Read the model definition and answer for the solid it produces. Units are mm, in the model's axes. A direction names the side the tool comes from. Coordinates: 2 decimals unless noted, no trailing zeros. Write each loop counter-clockwise with the first axis right and the second up, starting at its lowest first coordinate (ties: lowest second). Pieces come first, ordered by that corner, then holes. Notation, with made-up numbers: (-1, 23) -> (31, 23) arc R34 ccw to (31, 57) -> close; hole circle Ø1 at (37.25, 65.5). An arc over 180 degrees is marked (long way). Return JSON: item names as keys, results as strings.
Autodesk Inventor part; units mm, degrees
ref_plane "CP1_XY" through (0, 0, -77.4) normal (0, 0, -1) x (1, 0, 0)
ref_plane "CP1_YZ" through (0, 0, -77.4) normal (1, 0, 0) x (0, -1, 0)
ref_plane "CP1_ZX" through (0, 0, -77.4) normal (0, -1, 0) x (0, 0, -1)
sketch "Sketch_1" plane through (0, 0, 0) normal (1, 0, 0) x (0, 1, 0)
  line L0 (0, -77.4) -> (0, 0)
  line L1 (0, 0) -> (3, 0)
  line L2 (3, 0) -> (3, -72.4)
  line L3 (3, -72.4) -> (8, -72.4)
  line L4 (8, -72.4) -> (8, -77.4)
  line L5 (8, -77.4) -> (0, -77.4)
  line L6 (0, -77.4) -> (0, 0)
revolve "Revolution1" add sketch "Sketch_1" angle 360 about axis through (0, 0, -77.4) along (0, 0, -1)
sketch "Sketch_2" plane through (0, 0, 0) normal (1, 0, 0) x (0, 1, 0)
  line L0 (0, 0) -> (0, 12)
  line L1 (0, 12) -> (2.3865, 12)
  line L2 (2.3865, 12) -> (3, 11.3865)
  line L3 (3, 11.3865) -> (3, 2.2222)
  line L4 (3, 2.2222) -> (2.0586, 1.2808)
  arc A0 (2.0586, 1.2808) -> (2, 1.1394) centre (2.2, 1.1394) ccw
  line L5 (2, 1.1394) -> (2, 0.2)
  arc A1 (2, 0.2) -> (2.2, 0) centre (2.2, 0.2) ccw
  line L6 (2.2, 0) -> (0, 0)
  line L7 (0, 0) -> (0, 12)
revolve "Revolution2" add sketch "Sketch_2" angle 360 about axis through (0, 0, 0) along (0, 0, -1)
thread "Thread1"
sketch "Sketch_8" plane through (0, 0, 0) normal (0, 0, 1) x (1, 0, 0)
  line L0 (-4.5, 5) -> (-4.5, -5)
  line L1 (-4.5, -5) -> (4.5, -5)
  line L2 (4.5, -5) -> (4.5, 5)
  line L3 (4.5, 5) -> (-4.5, 5)
  line L4 (-2.5, -4) -> (2.5, -4)
  line L5 (2.5, -4) -> (2.5, 4)
  line L6 (2.5, 4) -> (-2.5, 4)
  line L7 (-2.5, 4) -> (-2.5, -4)
extrude "Extrusion1" cut sketch "Sketch_8" against normal blind 3
ref_plane "CP1_XY" through (0, 0, -77.4) normal (0, 0, -1) x (1, 0, 0)
ref_plane "CP1_YZ" through (0, 0, -77.4) normal (1, 0, 0) x (0, -1, 0)
ref_plane "CP1_ZX" through (0, 0, -77.4) normal (0, -1, 0) x (0, 0, -1)
ref_plane "CP_P_XY" through (0, 0, -77.4) normal (0, 0, 1) x (1, 0, 0)
ref_plane "CP_P_YZ" through (0, 0, -77.4) normal (1, 0, 0) x (0, 1, 0)
ref_plane "CP_P_ZX" through (0, 0, -77.4) normal (0, 1, 0) x (0, 0, 1)
ref_plane "CP_PL_XY" through (0, 0, -3) normal (0, 0, 1) x (1, 0, 0)
ref_plane "CP_PL_YZ" through (0, 0, -3) normal (1, 0, 0) x (0, 1, 0)
ref_plane "CP_PL_ZX" through (0, 0, -3) normal (0, 1, 0) x (0, 0, 1)
ref_plane "DIM_ZM_XY" through (0, 3, -150) normal (1, 0, 0) x (0, 0, -1)
ref_plane "DIM_ZM_YZ" through (0, 3, -150) normal (0, 0, -1) x (0, 1, 0)
ref_plane "DIM_ZM_ZX" through (0, 3, -150) normal (0, 1, 0) x (1, 0, 0)
ref_plane "DISC_XY" through (0, 0, 5) normal (0, 0, -1) x (1, 0, 0)
ref_plane "DISC_YZ" through (0, 0, 5) normal (1, 0, 0) x (0, -1, 0)
ref_plane "DISC_ZX" through (0, 0, 5) normal (0, -1, 0) x (0, 0, -1)
ref_plane "NUT_6_10_T_1_XY" through (0, 0, -161) normal (0, 0, 1) x (1, 0, 0)
ref_plane "NUT_6_10_T_1_YZ" through (0, 0, -161) normal (1, 0, 0) x (0, 1, 0)
ref_plane "NUT_6_10_T_1_ZX" through (0, 0, -161) normal (0, 1, 0) x (0, 0, 1)
ref_plane "NUT_6_10_T_2_XY" through (0, 0, -158.8) normal (0, 0, 1) x (1, 0, 0)
ref_plane "NUT_6_10_T_2_YZ" through (0, 0, -158.8) normal (1, 0, 0) x (0, 1, 0)
ref_plane "NUT_6_10_T_2_ZX" through (0, 0, -158.8) normal (0, 1, 0) x (0, 0, 1)
ref_plane "NUT_CP_6_10_1_XY" through (0, 0, 10) normal (0, 0, 1) x (1, 0, 0)
ref_plane "NUT_CP_6_10_1_YZ" through (0, 0, 10) normal (1, 0, 0) x (0, 1, 0)
ref_plane "NUT_CP_6_10_1_ZX" through (0, 0, 10) normal (0, 1, 0) x (0, 0, 1)
ref_plane "NUT_CP_6_10_2_XY" through (0, 0, 7.8) normal (0, 0, 1) x (1, 0, 0)
ref_plane "NUT_CP_6_10_2_YZ" through (0, 0, 7.8) normal (1, 0, 0) x (0, 1, 0)
ref_plane "NUT_CP_6_10_2_ZX" through (0, 0, 7.8) normal (0, 1, 0) x (0, 0, 1)
properties part number "4186566 DPDM-50---(r)" material "Stainless Steel"
1. Flat-ended cylindrical pins translate along their axes: pin 1 Ø0.9 at (y, z) = (0, -2) entering from +X; pin 2 Ø8 at (y, z) = (-1, -3) entering from +X; pin 3 Ø6 at (x, z) = (1, -54) entering from -Y. Find the tip coordinate at first contact, or state that the pin passes through.
Taken from the geometry:
{"pin 1": "stops at x = 2.5", "pin 2": "stops at x = 3", "pin 3": "stops at y = -3"}
2. The part is cut by section D-D (x = -5.75). Determine the outline of the cut face in (y, z), then the cut area to 3 significant figures.
Taken from the geometry:
{"outline": "(-5.56, -77.4) -> (5.56, -77.4) -> (5.56, -72.4) -> (-5.56, -72.4) -> close", "area": "55.6 mm2"}
3. Consider L1, parallel to Z at x = 1.75, y = 3.75; L2, parallel to X at y = 0, z = -9; L3, parallel to X at y = -2, z = -33.5. Determine where each line is inside the solid, lowest interval first.
Taken from the geometry:
{"L1": "z = -77.4 to -72.4", "L2": "x = -3 to 3", "L3": "x = -2.24 to 2.24"}
4. The part is cut by section B-B (x = 0). Determine the outline of the cut face in (y, z), then the cut area to 3 significant figures.
Taken from the geometry:
{"outline": "(-8, -77.4) -> (8, -77.4) -> (8, -72.4) -> (3, -72.4) -> (3, 0) -> (2.2, 0) arc R0.2 cw to (2, 0.2) -> (2, 1.14) arc R0.2 cw to (2.06, 1.28) -> (3, 2.22) -> (3, 11.39) -> (2.39, 12) -> (-2.39, 12) -> (-3, 11.39) -> (-3, 2.22) -> (-2.06, 1.28) arc R0.2 cw to (-2, 1.14) -> (-2, 0.2) arc R0.2 cw to (-2.2, 0) -> (-3, 0) -> (-3, -72.4) -> (-8, -72.4) -> close", "area": "583 mm2"}
5. The part is cut by section A-A (y = 0). Determine the outline of the cut face in (x, z).
Taken from the geometry:
{"outline": "(-8, -77.4) -> (8, -77.4) -> (8, -72.4) -> (3, -72.4) -> (3, -3) -> (2.5, -3) -> (2.5, 0) -> (2.2, 0) arc R0.2 cw to (2, 0.2) -> (2, 1.14) arc R0.2 cw to (2.06, 1.28) -> (3, 2.22) -> (3, 11.39) -> (2.39, 12) -> (-2.39, 12) -> (-3, 11.39) -> (-3, 2.22) -> (-2.06, 1.28) arc R0.2 cw to (-2, 1.14) -> (-2, 0.2) arc R0.2 cw to (-2.2, 0) -> (-2.5, 0) -> (-2.5, -3) -> (-3, -3) -> (-3, -72.4) -> (-8, -72.4) -> close"}
6. For a pull along Z with two mould halves and no side action, classify faces 1 (the face through (-1.952, -0.434, 0.663)), 2 (the face through (0, -3, -37)), 3 (the face through (0, 0, -77.4)) as +Z half, -Z half, draft (parallel to the pull), parting line (faces both ways), or undercut.
Taken from the geometry:
{"face 1": "undercut", "face 2": "draft", "face 3": "-Z half"}
7. A tool of negligible diameter and unlimited length cuts with its end or side. For faces 4 (the face through (0.1, 3.4, -72.4)), 5 (the face through (2.3, 0.6, 0)), 6 (the face through (2.5, 0, -1)), from which of +Z, -Z, +X, -X, +Y, -Y can it reach the whole face along a straight path? Write none if from no direction.
Taken from the geometry:
{"face 4": "+Z", "face 5": "none", "face 6": "+X, +Y, -Y"}
8. The part is cut by section C-C (z = -22). Determine the outline of the cut face in (x, y), then the cut area to 3 significant figures.
Taken from the geometry:
{"outline": "circle Ø6 at (0, 0)", "area": "28.3 mm2"}
